For this review, take the finished solid that the model builds, in its own axes (mm). A direction names the side the tool comes from. Coordinates: 2 decimals unless noted, no trailing zeros. Loops run counter-clockwise (first coordinate to the right, second up) from the corner with the lowest first, then second, coordinate; pieces in that order, holes last. Notation, with made-up numbers: M 9.25,51.25 L 61.25,51.25 A14 ccw 61.25,70.25 Z; hole C 69.25,33 d11. An arc over 180 degrees is marked long. Put each result on its own line as item: value.
```python
from build123d import *

# Parameters (mm, degrees)
SKETCH_3_W          = 60
SKETCH_3_H          = 60
EXTRUDE_1_DEPTH     = 15
SKETCH_4_W          = 47.15
SKETCH_4_H          = 47.15
CUT_EXTRUDE_1_DEPTH = 12
SKETCH_5_R          = 1.325
CUT_EXTRUDE_2_DEPTH = 69.738635424
EXTRUDE_2_REACH     = 47
SKETCH_6_W          = 4
SKETCH_6_H          = 14.375
FILLET_1_R          = 8
SKETCH_11_R         = 1.75
CUT_EXTRUDE_5_DEPTH = 5.5
SKETCH_12_R         = 1.4
CUT_EXTRUDE_6_DEPTH = 5.5
SKETCH_13_W         = 10
SKETCH_13_H         = 5
EXTRUDE_3_DEPTH     = 4
CHAMFER_1_SIZE      = 0.5
SKETCH_15_W         = 12
SKETCH_15_H         = 12
CUT_EXTRUDE_7_DEPTH = 47.904157598
FILLET_2_R          = 2


with BuildPart() as part:
    # 草图3 → 凸台-拉伸1 (new body)
    with BuildSketch(Plane.XY):
        Rectangle(SKETCH_3_W, SKETCH_3_H)
    extrude(amount=EXTRUDE_1_DEPTH)

    # 草图4 → 切除-拉伸1 (cut)
    with BuildSketch(Plane.XY.offset(15)):
        Rectangle(SKETCH_4_W, SKETCH_4_H)
    extrude(amount=-CUT_EXTRUDE_1_DEPTH, mode=Mode.SUBTRACT)

    # 草图5 → 切除-拉伸2 (cut, through all)
    with BuildSketch(Plane.ZY.offset(30)):
        with Locations(Location((9.8, 6.025, 0), (0, 0, 270))):
            Circle(SKETCH_5_R)
        with Locations(Location((9.8, -6.025, 0), (0, 0, 270))):
            Circle(SKETCH_5_R)
    extrude(amount=-CUT_EXTRUDE_2_DEPTH, mode=Mode.SUBTRACT)

    # 草图6 → 凸台-拉伸2 (add, up to next)
    with BuildSketch(Plane.XY.offset(15), mode=Mode.PRIVATE) as extrude_2_sk1:
        with Locations((-21.575, 16.3875)):
            Rectangle(SKETCH_6_W, SKETCH_6_H)
    extrude_2_tool1 = extrude(extrude_2_sk1.sketch, amount=-EXTRUDE_2_REACH, mode=Mode.PRIVATE) - part.part
    # 草图6 → 凸台-拉伸2 (add, up to next)
    with BuildSketch(Plane.XY.offset(15), mode=Mode.PRIVATE) as extrude_2_sk2:
        with Locations((21.575, 16.3875)):
            Rectangle(SKETCH_6_W, SKETCH_6_H)
    extrude_2_tool2 = extrude(extrude_2_sk2.sketch, amount=-EXTRUDE_2_REACH, mode=Mode.PRIVATE) - part.part
    # 草图6 → 凸台-拉伸2 (add, up to next)
    with BuildSketch(Plane.XY.offset(15), mode=Mode.PRIVATE) as extrude_2_sk3:
        with Locations((21.575, -16.3875)):
            Rectangle(SKETCH_6_W, SKETCH_6_H)
    extrude_2_tool3 = extrude(extrude_2_sk3.sketch, amount=-EXTRUDE_2_REACH, mode=Mode.PRIVATE) - part.part
    # 草图6 → 凸台-拉伸2 (add, up to next)
    with BuildSketch(Plane.XY.offset(15), mode=Mode.PRIVATE) as extrude_2_sk4:
        with Locations((-21.575, -16.3875)):
            Rectangle(SKETCH_6_W, SKETCH_6_H)
    extrude_2_tool4 = extrude(extrude_2_sk4.sketch, amount=-EXTRUDE_2_REACH, mode=Mode.PRIVATE) - part.part
    add(extrude_2_tool1.solids().sort_by_distance((-21.575, 16.3875, 15))[0])
    add(extrude_2_tool2.solids().sort_by_distance((21.575, 16.3875, 15))[0])
    add(extrude_2_tool3.solids().sort_by_distance((21.575, -16.3875, 15))[0])
    add(extrude_2_tool4.solids().sort_by_distance((-21.575, -16.3875, 15))[0])

    # 圆角1
    fillet_1_edges = [part.edges().sort_by_distance(p)[0] for p in [
        (30, -30, 7.5),
        (-30, -30, 7.5),
    ]]
    fillet(fillet_1_edges, radius=FILLET_1_R)

    # 草图11 → 切除-拉伸5 (cut)
    with BuildSketch(Plane(origin=(0, 30, 0), x_dir=(1, 0, 0), z_dir=(0, 1, 0))):
        with Locations(Location((-17.5, -7.5, 0), (0, 0, 270))):
            Circle(SKETCH_11_R)
        with Locations(Location((17.5, -7.5, 0), (0, 0, 90))):
            Circle(SKETCH_11_R)
    extrude(amount=-CUT_EXTRUDE_5_DEPTH, mode=Mode.SUBTRACT)

    # 草图12 → 切除-拉伸6 (cut)
    with BuildSketch(Plane.XZ.offset(30)):
        with Locations(Location((-17.5, 7.5, 0), (0, 0, 270))):
            Circle(SKETCH_12_R)
        with Locations(Location((17.5, 7.5, 0), (0, 0, 90))):
            Circle(SKETCH_12_R)
    extrude(amount=-CUT_EXTRUDE_6_DEPTH, mode=Mode.SUBTRACT)

    # 草图13 → 凸台-拉伸3 (add)
    with BuildSketch(Plane(origin=(0, 30, 0), x_dir=(1, 0, 0), z_dir=(0, 1, 0))):
        with Locations((0, -7.5)):
            Rectangle(SKETCH_13_W, SKETCH_13_H)
    extrude(amount=EXTRUDE_3_DEPTH)

    # 倒角1
    chamfer_1_edges = [part.edges().sort_by_distance(p)[0] for p in [
        (5, 34, 7.5),
        (0, 34, 5),
        (-5, 34, 7.5),
        (0, 34, 10),
    ]]
    chamfer(chamfer_1_edges, length=CHAMFER_1_SIZE)

    # 草图15 → 切除-拉伸7 (cut, through all)
    with BuildSketch(Plane.XY.offset(3)):
        with Locations((4.275, -12.55)):
            Rectangle(SKETCH_15_W, SKETCH_15_H)
    extrude(amount=-CUT_EXTRUDE_7_DEPTH, mode=Mode.SUBTRACT)

    # 圆角2
    fillet_2_edges = [part.edges().sort_by_distance(p)[0] for p in [
        (-1.725, -18.55, 1.5),
        (-1.725, -6.55, 1.5),
        (10.275, -6.55, 1.5),
        (10.275, -18.55, 1.5),
    ]]
    fillet(fillet_2_edges, radius=FILLET_2_R)


solid = part.part
```
(1) Tool access review of faces 5 (the flat face through (-23.575, 0, 9)), 6 (the flat face through (0, 32, 10)), 7 (the flat face through (0, 32, 5)), 8 (the flat face through (-17, 24.5, 7)), 9 (the cylindrical face through (-1.1, -7.1, 1.5)): name each direction out of +Z, -Z, +X, -X, +Y, -Y from which nothing blocks a thin tool from reaching the whole face with its end or side.
Determined:
face 5: +Z
face 6: +Z, +X, -X, +Y
face 7: -Z, +X, -X, +Y
face 8: +Y
face 9: +Z, -Z
(2) Wall thickness on line 1 along X through (y, z) = (26, 7.75); line 2 along Y through (x, z) = (8, 2.5); line 3 along Y through (x, z) = (-11.5, 8.75) (3 decimals): over which ranges is each line inside the solid? List them lowest first. Write a range as [from, to].
Determined:
line 1: x = [-30, -19.23], [-15.77, 15.77], [19.23, 30]
line 2: y = [-30, -18.55], [-6.55, 30]
line 3: y = [-30, -23.575], [23.575, 30]
(3) Add section A-A (y = 28). Write out the cut boundary in (x, z).
Determined:
outline: M -30,0 L 30,0 L 30,15 L -30,15 Z; hole C -17.5,7.5 d3.5; hole C 17.5,7.5 d3.5
(4) Draft analysis for pull direction X (two halves, no side actions). For faces 1 (the flat face through (-22, -9.2, 9)), 2 (the flat face through (0, -30, 7)), 3 (the cylindrical face through (15.765, 27.288, 7.728)), 4 (the flat face through (-30, 4, 7)), state which applies: +X half, -X half, draft (parallel to the pull), parting line (faces both ways), or undercut.
Determined:
face 1: undercut
face 2: draft
face 3: undercut
face 4: -X half
(5) Add section D-D (y = -5.5). Write out the cut boundary in (x, z) (3 decimals), plus the area to 3 significant figures.
Determined:
outline: M -30,0 L 30,0 L 30,8.583 L 23.575,8.583 L 23.575,3 L -23.575,3 L -23.575,8.583 L -30,8.583 Z; M -30,11.017 L -23.575,11.017 L -23.575,15 L -30,15 Z; M 23.575,11.017 L 30,11.017 L 30,15 L 23.575,15 Z
area: 303 mm^2
(6) For pin 1 (4 mm diameter, centred on x = -15.5, y = 4.5, fed in from +Z); pin 2 (1 mm diameter, centred on y = 31, z = 8, fed in from +X); pin 3 (1.5 mm diameter, centred on x = 4, z = 2, fed in from +Y), all flat-tipped, find the tip position at first contact; note any pin that passes through.
Determined:
pin 1: stops at z = 3
pin 2: stops at x = 5
pin 3: stops at y = 30
(7) Add section C-C (z = 13). Write out the cut boundary in (x, y) (3 decimals).
Determined:
outline: M -30,-22 A8 ccw -22,-30 L 22,-30 A8 ccw 30,-22 L 30,30 L -30,30 Z; hole M -23.575,-9.2 L -19.575,-9.2 L -19.575,-23.575 L 19.575,-23.575 L 19.575,-9.2 L 23.575,-9.2 L 23.575,9.2 L 19.575,9.2 L 19.575,23.575 L -19.575,23.575 L -19.575,9.2 L -23.575,9.2 Z
(8) Add section B-B (x = -17.5). Write out the cut boundary in (y, z) (3 decimals).
Determined:
outline: M -30,0 L 30,0 L 30,5.75 L 24.5,5.75 L 24.5,9.25 L 30,9.25 L 30,15 L 23.575,15 L 23.575,3 L -23.575,3 L -23.575,15 L -30,15 L -30,8.9 L -24.5,8.9 L -24.5,6.1 L -30,6.1 Z
